```python
from build123d import *

# Parameters (mm, degrees)
SKETCH_1_W          = 71.5
SKETCH_1_H          = 152.8
EXTRUDE_1_DEPTH     = 8.2
FILLET_3_R          = 3.5
FILLET_4_R          = 3.5
FILLET_5_R          = 3.5
FILLET_6_R          = 3.5
EXTRUDE_3_DEPTH     = 0.8
EXTRUDE_4_DEPTH     = 0.8
SKETCH_5_W          = 42
SKETCH_5_H          = 42
EXTRUDE_5_DEPTH     = 1.5
FILLET_10_R         = 3.5
FILLET_11_R         = 3.5
FILLET_12_R         = 3.5
FILLET_13_R         = 3.5
CUT_EXTRUDE_1_DEPTH = 10
SKETCH_7_W          = 6
SKETCH_7_H          = 0.5
EXTRUDE_6_DEPTH     = 8
SKETCH_8_R          = 1.25
CUT_EXTRUDE_2_DEPTH = 10
CUT_EXTRUDE_3_DEPTH = 10
SKETCH_13_W         = 35
SKETCH_13_H         = 35
EXTRUDE_7_DEPTH     = 1.5
FILLET_14_R         = 3.5
CUT_EXTRUDE_4_DEPTH = 10


with BuildPart() as part:
    # 草图1 → 凸台-拉伸1 (new body)
    with BuildSketch(Plane.XY):
        Rectangle(SKETCH_1_W, SKETCH_1_H)
    extrude(amount=EXTRUDE_1_DEPTH)

    # 圆角3
    fillet_3_edges = [part.edges().sort_by_distance(p)[0] for p in [
        (-35.75, 76.4, 4.1),
    ]]
    fillet(fillet_3_edges, radius=FILLET_3_R)

    # 圆角4
    fillet_4_edges = [part.edges().sort_by_distance(p)[0] for p in [
        (35.75, 76.4, 4.1),
    ]]
    fillet(fillet_4_edges, radius=FILLET_4_R)

    # 圆角5
    fillet_5_edges = [part.edges().sort_by_distance(p)[0] for p in [
        (35.75, -76.4, 4.1),
    ]]
    fillet(fillet_5_edges, radius=FILLET_5_R)

    # 圆角6
    fillet_6_edges = [part.edges().sort_by_distance(p)[0] for p in [
        (-35.75, -76.4, 4.1),
    ]]
    fillet(fillet_6_edges, radius=FILLET_6_R)

    # 草图3 → 凸台-拉伸3 (add)
    with BuildSketch(Plane(origin=(35.75, 0, 0), x_dir=(0, 0, -1), z_dir=(1, 0, 0))):
        with BuildLine():
            Line((-5.499995889, 43.056517333), (-5.499995889, 21.056517333))
            ThreePointArc((-5.499995889, 21.056517333), (-4.142644, 19.672279908), (-2.703526658, 20.971302108))
            Line((-2.703526658, 20.971302108), (-2.703526658, 42.915947634))
            ThreePointArc((-2.703526658, 42.915947634), (-4.029693086, 44.419944517), (-5.499995889, 43.056517333))
        make_face()
    extrude(amount=EXTRUDE_3_DEPTH)

    # 草图4 → 凸台-拉伸4 (add)
    with BuildSketch(Plane(origin=(35.75, 0, 0), x_dir=(0, 0, -1), z_dir=(1, 0, 0))):
        with BuildLine():
            Line((-5.5, 14), (-5.5, 2))
            ThreePointArc((-5.5, 2), (-4.1, 0.6), (-2.7, 2))
            Line((-2.7, 2), (-2.7, 14))
            ThreePointArc((-2.7, 14), (-4.1, 15.4), (-5.5, 14))
        make_face()
    extrude(amount=EXTRUDE_4_DEPTH)

    # 草图5 → 凸台-拉伸5 (add)
    with BuildSketch(Plane(origin=(0, 0, 0), x_dir=(-1, 0, 0), z_dir=(0, 0, -1))):
        with Locations((-12, 52)):
            Rectangle(SKETCH_5_W, SKETCH_5_H)
    extrude(amount=EXTRUDE_5_DEPTH)

    # 圆角10
    fillet_10_edges = [part.edges().sort_by_distance(p)[0] for p in [
        (33, 73, -0.75),
    ]]
    fillet(fillet_10_edges, radius=FILLET_10_R)

    # 圆角11
    fillet_11_edges = [part.edges().sort_by_distance(p)[0] for p in [
        (-9, 73, -0.75),
    ]]
    fillet(fillet_11_edges, radius=FILLET_11_R)

    # 圆角12
    fillet_12_edges = [part.edges().sort_by_distance(p)[0] for p in [
        (33, 31, -0.75),
    ]]
    fillet(fillet_12_edges, radius=FILLET_12_R)

    # 圆角13
    fillet_13_edges = [part.edges().sort_by_distance(p)[0] for p in [
        (-9, 31, -0.75),
    ]]
    fillet(fillet_13_edges, radius=FILLET_13_R)

    # 草图6 → 切除-拉伸1 (cut)
    with BuildSketch(Plane(origin=(0, -76.4, 0), x_dir=(-1, 0, 0), z_dir=(0, -1, 0))):
        with BuildLine():
            Line((3, -6.35), (-3, -6.35))
            ThreePointArc((-3, -6.35), (-4.060660172, -5.910660172), (-4.5, -4.85))
            Line((-4.5, -4.85), (-4.5, -3.35))
            ThreePointArc((-4.5, -3.35), (-4.060660172, -2.289339828), (-3, -1.85))
            Line((-3, -1.85), (3, -1.85))
            ThreePointArc((3, -1.85), (4.060660172, -2.289339828), (4.5, -3.35))
            Line((4.5, -3.35), (4.5, -4.85))
            ThreePointArc((4.5, -4.85), (4.060660172, -5.910660172), (3, -6.35))
        make_face()
    extrude(amount=-CUT_EXTRUDE_1_DEPTH, mode=Mode.SUBTRACT)

    # 草图7 → 凸台-拉伸6 (add)
    with BuildSketch(Plane(origin=(0, -66.4, 0), x_dir=(-1, 0, 0), z_dir=(0, -1, 0))):
        with Locations((0, -4.1)):
            Rectangle(SKETCH_7_W, SKETCH_7_H)
    extrude(amount=EXTRUDE_6_DEPTH)

    # 草图8 → 切除-拉伸2 (cut)
    with BuildSketch(Plane(origin=(0, -76.4, 0), x_dir=(-1, 0, 0), z_dir=(0, -1, 0))):
        with Locations(Location((-9.942250917, -4.1, 0), (0, 0, 90))):
            Circle(SKETCH_8_R)
        with Locations(Location((-12.942250917, -4.1, 0), (0, 0, 90))):
            Circle(SKETCH_8_R)
        with Locations(Location((-15.942250917, -4.1, 0), (0, 0, 90))):
            Circle(SKETCH_8_R)
        with Locations(Location((-18.942250917, -4.1, 0), (0, 0, 90))):
            Circle(SKETCH_8_R)
        with Locations(Location((-21.942250917, -4.1, 0), (0, 0, 90))):
            Circle(SKETCH_8_R)
        with Locations(Location((-24.942250917, -4.1, 0), (0, 0, 90))):
            Circle(SKETCH_8_R)
        with Locations(Location((-27.942250917, -4.1, 0), (0, 0, 90))):
            Circle(SKETCH_8_R)
    extrude(amount=-CUT_EXTRUDE_2_DEPTH, mode=Mode.SUBTRACT)

    # 草图11 → 切除-拉伸3 (cut)
    with BuildSketch(Plane.XZ.offset(76.4)):
        with BuildLine():
            Line((-9.2, 5.1), (-8.8, 5.1))
            ThreePointArc((-8.8, 5.1), (-8.587867966, 5.012132034), (-8.5, 4.8))
            Line((-8.5, 4.8), (-8.5, 3.4))
            ThreePointArc((-8.5, 3.4), (-8.587867966, 3.187867966), (-8.8, 3.1))
            Line((-8.8, 3.1), (-9.2, 3.1))
            ThreePointArc((-9.2, 3.1), (-9.412132034, 3.187867966), (-9.5, 3.4))
            Line((-9.5, 3.4), (-9.5, 4.8))
            ThreePointArc((-9.5, 4.8), (-9.412132034, 5.012132034), (-9.2, 5.1))
        make_face()
    extrude(amount=-CUT_EXTRUDE_3_DEPTH, mode=Mode.SUBTRACT)

    # 草图13 → 凸台-拉伸7 (add)
    with BuildSketch(Plane(origin=(0, 0, -1.5), x_dir=(-1, 0, 0), z_dir=(0, 0, -1))):
        with Locations((-12, 52)):
            Rectangle(SKETCH_13_W, SKETCH_13_H)
    extrude(amount=EXTRUDE_7_DEPTH)

    # 圆角14
    fillet_14_edges = [part.edges().sort_by_distance(p)[0] for p in [
        (-5.5, 34.5, -2.25),
        (-5.5, 69.5, -2.25),
        (29.5, 69.5, -2.25),
        (29.5, 34.5, -2.25),
    ]]
    fillet(fillet_14_edges, radius=FILLET_14_R)

    # 草图14 → 切除-拉伸4 (cut)
    with BuildSketch(Plane(origin=(0, -76.4, 0), x_dir=(-1, 0, 0), z_dir=(0, -1, 0))):
        with BuildLine():
            Line((16.012447704, -2.550259118), (28.012447704, -2.64984418))
            ThreePointArc((28.012447704, -2.64984418), (29.499948351, -4.162240235), (27.987552296, -5.649740882))
            Line((27.987552296, -5.649740882), (15.987552296, -5.55015582))
            ThreePointArc((15.987552296, -5.55015582), (14.500051649, -4.037759765), (16.012447704, -2.550259118))
        make_face()
    extrude(amount=-CUT_EXTRUDE_4_DEPTH, mode=Mode.SUBTRACT)


solid = part.part
```
CAD build for the part. Positions are in the model's coordinates, mm. A direction names the side the tool comes from. Round coordinates to 2 decimals unless told otherwise and drop trailing zeros. Loops run counter-clockwise (first coordinate to the right, second up) from the corner with the lowest first, then second, coordinate; pieces in that order, holes last. Notation, with made-up numbers: M 5,-22.5 L 23,-22.5 A30 cw 23,1.5 Z; hole C 2,39.25 d2. An arc over 180 degrees is marked long. Use a Markdown table: item, result. Add a question column.
(1) Which spindle directions (+Z, -Z, +X, -X, +Y, -Y) get a long thin tool onto all of the face, cutting with end or side? Do faces 1 (the face through (0, 76.4, 4)), 2 (the face through (-7.95, 72, -0.76)), 3 (the face through (-35.75, -1, 4)), 4 (the face through (31, 52, -1.5)), 5 (the face through (0, -70, 3.85)). Say none if no direction does.
(2) Cut at B-B (y = -60). Give the cut face in (x, z), and give its area (3 significant figures).
(3) Pull direction X, two halves, no side cores. Call faces 6 (the face through (-29.5, -71.5, 4.1)), 7 (the face through (0, -76.4, 1)), 8 (the face through (-4.45, 35.5, -2.26)): +X half, -X half, draft (parallel to the pull), parting line (faces both ways), or undercut.
(4) Cut at A-A (y = 49). Give the cut face in (x, z).
(5) Flat gauge pins, fed straight in: pin 1 (1.5 mm diameter, centred on y = -72, z = 4, fed in from +X); pin 2 (1.8 mm diameter, centred on x = 0.5, y = -71.5, fed in from -Z); pin 3 (0.8 mm diameter, centred on x = 18.5, z = -0.5, fed in from -Y). Where does each tip first touch, or does it go through?
(6) Drill centre lines: line 1 (Z direction, x = 16.5, y = -21); line 2 (Y direction, x = 17, z = -2.5); line 3 (Y direction, x = -17.5, z = 2.75). Where is each one in solid material? Low to high.
Geometry says:
| question | item | result |
|---|---|---|
| 1 | face 1 | +Z, -Z, +X, -X, +Y |
| 1 | face 2 | -Z, -X, +Y |
| 1 | face 3 | +Z, -Z, -X, +Y, -Y |
| 1 | face 4 | -Z |
| 1 | face 5 | -Y |
| 2 | outline | M -35.75,0 L 35.75,0 L 35.75,8.2 L -35.75,8.2 Z |
| 2 | area | 586 mm² |
| 3 | face 6 | undercut |
| 3 | face 7 | draft |
| 3 | face 8 | -X half |
| 4 | outline | M -35.75,0 L -9,0 L -9,-1.5 L -5.5,-1.5 L -5.5,-3 L 29.5,-3 L 29.5,-1.5 L 33,-1.5 L 33,0 L 35.75,0 L 35.75,8.2 L -35.75,8.2 Z |
| 5 | pin 1 | stops at x = 35.75 |
| 5 | pin 2 | stops at z = 0 |
| 5 | pin 3 | stops at y = 31 |
| 6 | line 1 | z = 0 to 8.2 |
| 6 | line 2 | y = 34.5 to 69.5 |
| 6 | line 3 | y = -66.4 to 76.4 |
